```python
from build123d import *

# Parameters (mm, degrees)
F0_W     = 64
F0_H     = 42.4
F0_R     = 1
F1_DEPTH = 2
F2_R     = 5


with BuildPart() as f1:
    # F0 (on Top) → F1 (new body)
    with BuildSketch(Plane.XY):
        Rectangle(F0_W, F0_H)
        with Locations((-9.9, 0)):
            Circle(F0_R, mode=Mode.SUBTRACT)
        with Locations((20.6, 0)):
            Circle(F0_R, mode=Mode.SUBTRACT)
    extrude(amount=F1_DEPTH)

    # F2
    f2_edges = [f1.edges().sort_by_distance(p)[0] for p in [
        (32, -21.2, 1),
        (32, 21.2, 1),
        (-32, 21.2, 1),
        (-32, -21.2, 1),
    ]]
    fillet(f2_edges, radius=F2_R)


solid = f1.part
```
Verification items for the finished model (mm, model axes). Give positions to 0.01 mm unless a question says otherwise; leave off trailing zeros. Order: outer loops, then holes, each group sorted by start corner. A loop starts at its lowest first (then second) coordinate and runs counter-clockwise, first axis right, second up. Notation, with made-up numbers: M 64.25,79 L 116.25,79 A4 cw 116.25,84 Z; hole C 77,82.25 d5. An arc over 180 degrees is marked long. Answer in a Markdown table with one row per item. Add a question column.
Item 1: Mould release check, pull along X, two halves, no side actions. Record for faces 1 (the cylindrical face through (-30.57, 19.7, 1.01)), 2 (the flat face through (0, 0, 0)), 3 (the cylindrical face through (19.6, 0, 1)): released by +X, released by -X, zero draft, split by the parting line, or undercut.
Item 2: Gauge pin test, flat ends, axial feed: pin 1 (3 mm diameter, centred on x = -21, y = -13.5, fed in from -Z); pin 2 (1.2 mm diameter, centred on x = 20.6, y = 0, fed in from +Z). Record the tip position at first contact, or that the pin passes through.
Item 3: Scan lines: probe 1 along Y at (x, z) = (20.6, 1.25); probe 2 along Y at (x, z) = (-9.5, 0.85); probe 3 along Y at (x, z) = (29, 1.15). Record each from-to range of solid material in increasing order. Write a range as from..to.
Item 4: Section check A-A, the plane y = 0. Enter the section's corners in (x, z).
Item 5: Section check B-B, the plane x = 20.6. Enter the section's corners in (y, z).
Filled sheet:
| question | item | result |
|---|---|---|
| 1 | face 1 | released by -X |
| 1 | face 2 | zero draft |
| 1 | face 3 | undercut |
| 2 | pin 1 | stops at z = 0 |
| 2 | pin 2 | passes through |
| 3 | probe 1 | y = -21.2..-1, 1..21.2 |
| 3 | probe 2 | y = -21.2..-0.92, 0.92..21.2 |
| 3 | probe 3 | y = -20.78..20.78 |
| 4 | outline | M -32,0 L -10.9,0 L -10.9,2 L -32,2 Z; M -8.9,0 L 19.6,0 L 19.6,2 L -8.9,2 Z; M 21.6,0 L 32,0 L 32,2 L 21.6,2 Z |
| 5 | outline | M -21.2,0 L -1,0 L -1,2 L -21.2,2 Z; M 1,0 L 21.2,0 L 21.2,2 L 1,2 Z |
